Job drawing, mm, ordinate dimensions from the low corner. One solid piece. A direction names the side the tool comes from. Coordinates: 2 decimals unless noted, no trailing zeros. Loops run counter-clockwise (first coordinate to the right, second up) from the corner with the lowest first, then second, coordinate; pieces in that order, holes last. Notation, with made-up numbers: (0, -9) - (24, -9) arc R27 ccw to (24, 14) - close; hole circle Ø2 at (14.25, 28.5). An arc over 180 degrees is marked (long way). Use a Markdown table: item, result. Add a question column.
1. Band-saw the part on B-B, the plane z = 21. Give the cut face in (x, y).
2. Drop flat-ended pins along their axis: pin 1 (21 mm diameter, centred on y = 30.5, z = 15, fed in from -X); pin 2 (3 mm diameter, centred on y = 25, z = 6, fed in from +X); pin 3 (6 mm diameter, centred on y = 57.5, z = 5, fed in from -X). Give the stop position or say it passes through.
3. Band-saw the part on D-D, the plane y = 47. Give the cut face in (x, z), plus the area to 3 significant figures.
4. 3-axis set-ups, long thin cutter, end or side, ignore diameter. For the marked faces 1, 2, 3 and 4: which of +Z, -Z, +X, -X, +Y, -Y reach the whole face in a straight line?
5. Band-saw the part on A-A, the plane z = 37. Give the cut face in (x, y).
6. Pull direction Y, two halves, no side cores. Call the marked faces 5, 6, 7 and 8: pulls with the +Y half, pulls with the -Y half, needs draft (parallel to the pull), parting line crosses it, or undercut.
7. Wall check: probe 1 along Y at (x, z) = (14.5, 36); probe 2 along Y at (x, z) = (37.5, 4); probe 3 along X at (y, z) = (31, 3.5). Give the ranges that are in metal, low to high. Write a range as [from, to].
8. Band-saw the part on C-C, the plane x = 18.5. Give the cut face in (y, z), plus the area to 3 significant figures.
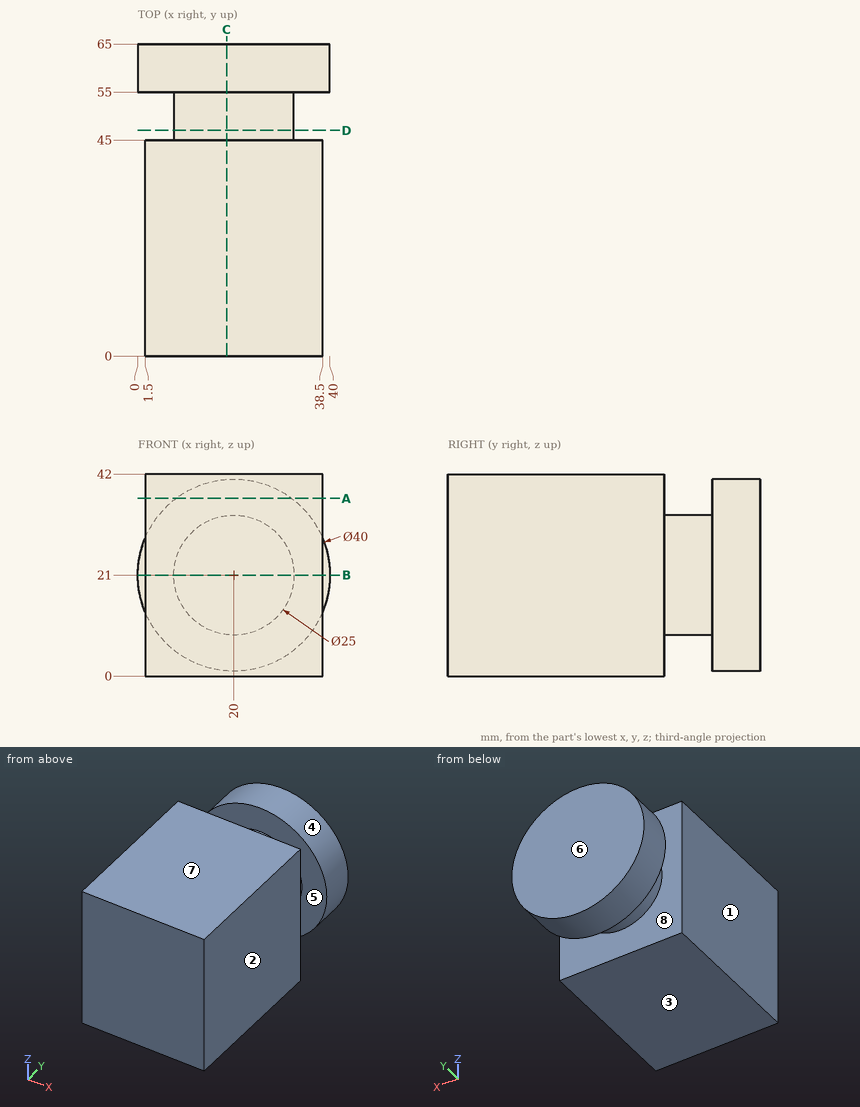
Geometry check:
| question | item | result |
|---|---|---|
| 1 | outline | (0, 55) - (7.5, 55) - (7.5, 45) - (1.5, 45) - (1.5, 0) - (38.5, 0) - (38.5, 45) - (32.5, 45) - (32.5, 55) - (40, 55) - (40, 65) - (0, 65) - close |
| 2 | pin 1 | stops at x = 1.5 |
| 2 | pin 2 | stops at x = 38.5 |
| 2 | pin 3 | stops at x = 4.8 |
| 3 | outline | circle Ø25 at (20, 21) |
| 3 | area | 491 mm^2 |
| 4 | face 1 | +Z, -Z, -X, -Y |
| 4 | face 2 | +Z, -Z, +X, -Y |
| 4 | face 3 | -Z, +X, -X, +Y, -Y |
| 4 | face 4 | +Y |
| 5 | outline | (1.5, 0) - (38.5, 0) - (38.5, 45) - (1.5, 45) - close; (8, 55) - (32, 55) - (32, 65) - (8, 65) - close |
| 6 | face 5 | undercut |
| 6 | face 6 | pulls with the +Y half |
| 6 | face 7 | needs draft |
| 6 | face 8 | undercut |
| 7 | probe 1 | y = [0, 45], [55, 65] |
| 7 | probe 2 | y = [0, 45] |
| 7 | probe 3 | x = [1.5, 38.5] |
| 8 | outline | (0, 0) - (45, 0) - (45, 8.59) - (55, 8.59) - (55, 1.06) - (65, 1.06) - (65, 40.94) - (55, 40.94) - (55, 33.41) - (45, 33.41) - (45, 42) - (0, 42) - close |
| 8 | area | 2,540 mm^2 |
